```python
from build123d import *

# Parameters (mm, degrees)
CROQUIS1_R                   = 22.5
CROQUIS2_R                   = 30
CROQUIS3_R                   = 30
SALIENTE_EXTRUIR1_DEPTH      = 105
CROQUIS4_R                   = 32
SALIENTE_EXTRUIR2_DEPTH      = 10
CROQUIS6_R                   = 23
CORTAR_EXTRUIR1_DEPTH        = 161
SALIENTE_EXTRUIR3_DEPTH      = 3
SALIENTE_EXTRUIR3_DEPTH_BACK = 5
CROQUIS7_R                   = 24
CROQUIS7_R_2                 = 23
REDONDEO1_R                  = 5
CROQUIS9_W                   = 12
CROQUIS9_H                   = 40
CORTAR_EXTRUIR2_DEPTH        = 525
SALIENTE_EXTRUIR4_START      = -15
SALIENTE_EXTRUIR4_DEPTH      = 15
SALIENTE_EXTRUIR5_DEPTH      = 10
CROQUIS12_R                  = 1.5
CORTAR_EXTRUIR3_DEPTH        = 13


with BuildPart() as part:
    # Croquis1 → Recubrir1 section 0
    with BuildSketch(Plane(origin=(0, 0, 0), x_dir=(1, 0, 0), z_dir=(0, 1, 0))):
        Circle(CROQUIS1_R)
    # Croquis2 → Recubrir1 section 1
    with BuildSketch(Plane(origin=(0, 9, 0), x_dir=(1, 0, 0), z_dir=(0, 1, 0))):
        Circle(CROQUIS2_R)
    loft()

    # Croquis3 → Saliente-Extruir1 (add)
    with BuildSketch(Plane(origin=(0, 9, 0), x_dir=(1, 0, 0), z_dir=(0, 1, 0))):
        with Locations(Location((0, 0, 0), (0, 0, 270))):
            Circle(CROQUIS3_R)
    extrude(amount=SALIENTE_EXTRUIR1_DEPTH)

    # Croquis4 → Saliente-Extruir2 (add)
    with BuildSketch(Plane(origin=(0, 114, 0), x_dir=(1, 0, 0), z_dir=(0, 1, 0))):
        with Locations(Location((0, 0, 0), (0, 0, 270))):
            Circle(CROQUIS4_R)
    extrude(amount=SALIENTE_EXTRUIR2_DEPTH)

    # Croquis6 → Cortar-Extruir1 (cut)
    with BuildSketch(Plane(origin=(0, 124, 0), x_dir=(1, 0, 0), z_dir=(0, 1, 0))):
        with Locations(Location((0, 0, 0), (0, 0, 270))):
            Circle(CROQUIS6_R)
    extrude(amount=-CORTAR_EXTRUIR1_DEPTH, mode=Mode.SUBTRACT)

    # Croquis7 → Saliente-Extruir3 (add, two sides: drawn at the far end of the back side and taken through both)
    with BuildSketch(Plane(origin=(0, 0, 0), x_dir=(1, 0, 0), z_dir=(0, 1, 0)).offset(-SALIENTE_EXTRUIR3_DEPTH_BACK)):
        with Locations(Location((0, 0, 0), (0, 0, 270))):
            Circle(CROQUIS7_R)
        with Locations(Location((0, 0, 0), (0, 0, 270))):
            Circle(CROQUIS7_R_2, mode=Mode.SUBTRACT)
    extrude(amount=SALIENTE_EXTRUIR3_DEPTH + SALIENTE_EXTRUIR3_DEPTH_BACK)

    # Redondeo1
    # the kernel refuses this fillet: 5 mm, written as the material it adds along each edge
    with BuildSketch(Plane(origin=(0, 114, 0), x_dir=(0, 0, 1), z_dir=(-1, 0, 0))) as redondeo1_piece_1:
        with BuildLine():
            CenterArc((35, -4), REDONDEO1_R, 126.869897646, 53.130102354)
            Line((32, 0), (30, 0))
            Line((30, 0), (30, -4))
        make_face()
    redondeo1_piece_1_solid = revolve(axis=Axis((0, 114, 0), (0, 1, 0)), mode=Mode.PRIVATE)
    add([redondeo1_piece_1_solid])
    # the kernel refuses this fillet: 5 mm, written as the material it takes off along each edge
    with BuildSketch(Plane(origin=(0, 9, 0), x_dir=(1, 0, 0), z_dir=(0, 0, 1))) as redondeo1_2_piece_1:
        with BuildLine():
            CenterArc((30 - REDONDEO1_R, REDONDEO1_R * 0.362049935181), REDONDEO1_R, 320.194428908, 39.805571092)
            Line((30, REDONDEO1_R * 0.362049935181), (30, 0))
            Line((30, 0), (30 - REDONDEO1_R * 0.231778720403, -REDONDEO1_R * 0.278134464483))
        make_face()
    redondeo1_2_piece_1_solid = revolve(axis=Axis((0, 9, 0), (0, 1, 0)), revolution_arc=270, mode=Mode.PRIVATE)
    with BuildSketch(Plane(origin=(0, 9, 0), x_dir=(0, 0, 1), z_dir=(-1, 0, 0))) as redondeo1_2_piece_2:
        with BuildLine():
            CenterArc((30 - REDONDEO1_R, REDONDEO1_R * 0.362049935181), REDONDEO1_R, 320.194428908, 39.805571092)
            Line((30, REDONDEO1_R * 0.362049935181), (30, 0))
            Line((30, 0), (30 - REDONDEO1_R * 0.231778720403, -REDONDEO1_R * 0.278134464483))
        make_face()
    redondeo1_2_piece_2_solid = revolve(axis=Axis((0, 9, 0), (0, 1, 0)), revolution_arc=90, mode=Mode.PRIVATE)
    add([redondeo1_2_piece_1_solid, redondeo1_2_piece_2_solid], mode=Mode.SUBTRACT)

    # Croquis9 → Cortar-Extruir2 (cut)
    with BuildSketch(Plane.XY):
        with Locations((-9, 84)):
            Rectangle(CROQUIS9_W, CROQUIS9_H)
    extrude(amount=-CORTAR_EXTRUIR2_DEPTH, mode=Mode.SUBTRACT)

    # Croquis10 → Saliente-Extruir4 (add)
    with BuildSketch(Plane(origin=(0, 84, 0), x_dir=(1, 0, 0), z_dir=(0, 1, 0)).offset(SALIENTE_EXTRUIR4_START)):
        with BuildLine():
            Line((0, -30), (0, -33.675648379))
            Line((0, -33.675648379), (30, -33.675648379))
            Line((30, -33.675648379), (30, -23.675648379))
            Line((30, -23.675648379), (23.549751452, -18.585187827))
            ThreePointArc((23.549751452, -18.585187827), (13.085189437, -26.995885194), (0, -30))
        make_face()
    extrude(amount=SALIENTE_EXTRUIR4_DEPTH)

    # Croquis11 → Saliente-Extruir5 (add)
    with BuildSketch(Plane(origin=(0, 24, 0), x_dir=(1, 0, 0), z_dir=(0, 1, 0))):
        with BuildLine():
            Line((30, -23.675648379), (23.549751452, -18.585187827))
            ThreePointArc((23.549751452, -18.585187827), (13.085189437, -26.995885194), (0, -30))
            Line((0, -30), (0, -33.675648379))
            Line((0, -33.675648379), (30, -33.675648379))
            Line((30, -33.675648379), (30, -23.675648379))
        make_face()
    extrude(amount=SALIENTE_EXTRUIR5_DEPTH)

    # Croquis12 → Cortar-Extruir3 (cut)
    with BuildSketch(Plane.XY.offset(33.675648379)):
        with Locations((15, 29)):
            Circle(CROQUIS12_R)
        with Locations((15, 76.5)):
            Circle(CROQUIS12_R)
    extrude(amount=-CORTAR_EXTRUIR3_DEPTH, mode=Mode.SUBTRACT)


solid = part.part
```
Work out the finished part from the listing and answer in its coordinate system (mm). A direction names the side the tool comes from. Coordinates: 2 decimals unless noted, no trailing zeros. Loops run counter-clockwise (first coordinate to the right, second up) from the corner with the lowest first, then second, coordinate; pieces in that order, holes last.
1) Section D-D (y = 51) is taken. Give the vertices of the cut face in (x, z).
Results:
outline: circle Ø60 at (0, 0); hole circle Ø46 at (0, 0)
2) Section B-B (y = 81) is taken. Give the vertices of the cut face in (x, z), plus the area to 3 significant figures.
Results:
outline: (-15, -25.98) - (-15, -17.44) arc R23 cw (long way) to (-3, -22.8) - (-3, -29.85) arc R30 ccw to (23.55, 18.59) - (30, 23.68) - (30, 33.68) - (0, 33.68) - (0, 30) arc R30 ccw to start
area: 1,320 mm2
3) For faces 1 (the flat face through (0, 29, 32)), 2 (the flat face through (-3, 84, -26)), 3 (the flat face through (18, 34, 29)), 4 (the cylindrical face through (13.89, 30.01, 27.27)), 5 (the flat face through (26.82, 28.93, 21.166)), determine the directions among +Z, -Z, +X, -X, +Y, -Y from which every point of the face is accessible in a straight line to the end or side of a thin tool.
Results:
face 1: +Z, -X, -Y
face 2: -Z
face 3: +Z, +X
face 4: +Z
face 5: +X, -Y
4) Consider probe 1 along X at (y, z) = (79.5, 0); probe 2 along Y at (x, z) = (15, 27); probe 3 along Y at (x, z) = (15, 28). Determine where each line is inside the solid, lowest interval first.
Results:
probe 1: x = -30 to -23, 23 to 30
probe 2: y = 24 to 27.5, 30.5 to 34, 69 to 75, 78 to 84, 112.84 to 124
probe 3: y = 24 to 27.5, 30.5 to 34, 69 to 75, 78 to 84, 113.81 to 124
5) For a pull along X with two mould halves and no side action, classify faces 6 (the flat face through (18, 84, 29)), 7 (the flat face through (15, 77, 20.676)), 8 (the flat face through (30, 76, 29)), 9 (the cylindrical face through (-18, 60, -24)) as +X half, -X half, draft (parallel to the pull), parting line (faces both ways), or undercut.
Results:
face 6: draft
face 7: undercut
face 8: +X half
face 9: parting line
6) Section C-C (x = -8) is taken. Give the number of separate pieces and of enclosed holes in the cut face, plus the area to 3 significant figures.
Results:
separate pieces: 3
enclosed holes: 0
area: 1,520 mm2
7) Section A-A (y = 29) is taken. Give the vertices of the cut face in (x, z), plus the area to 3 significant figures.
Results:
outline: (0, 30) arc R30 ccw (long way) to (23.55, 18.59) - (30, 23.68) - (30, 33.68) - (16.5, 33.68) - (16.5, 20.68) - (13.5, 20.68) - (13.5, 33.68) - (0, 33.68) - close; hole circle Ø46 at (0, 0)
area: 1,380 mm2
8) Flat-ended cylindrical pins translate along their axes: pin 1 (1 mm diameter, centred on y = 58.5, z = 18, fed in from +X); pin 2 (2 mm diameter, centred on y = 52, z = -22, fed in from +X); pin 3 (2 mm diameter, centred on x = -19, z = -22.5, fed in from -Y); pin 4 (12 mm diameter, centred on x = 15.5, z = 29, fed in from +Y). Find the tip coordinate at first contact, or state that the pin passes through.
Results:
pin 1: stops at x = 24.37
pin 2: stops at x = 21.42
pin 3: stops at y = 7.14
pin 4: stops at y = 124
